Source: three-view drawing plus pictorial views. Frame: mm from the lowest corner of the part. A direction names the side the tool comes from. Coordinates: 2 decimals unless noted, no trailing zeros. Write each loop counter-clockwise with the first axis right and the second up, starting at its lowest first coordinate (ties: lowest second). Pieces come first, ordered by that corner, then holes. Notation, with made-up numbers: (10.5, -20) - (47.5, -20) arc R6 cw to (47.5, -14) - close; hole circle Ø4 at (22, 85.5). An arc over 180 degrees is marked (long way). Answer as a JSON object with one key per item and string values. Group by question number.
Item 1: Section C-C on y = 10. Return loops of the section in (x, z), and give its area (3 significant figures).
Item 2: Line query: line 1 along X through (y, z) = (13.75, 10.5); line 2 along X through (y, z) = (11.75, 22.75); line 3 along Y through (x, z) = (7.5, 10). Output: solid intervals per line, ascending. Write a range as from..to.
Item 3: Section D-D on x = 27.5. Return loops of the section in (y, z).
Item 4: Section A-A on z = 10.5. Return loops of the section in (x, y), and give its area (3 significant figures).
Item 5: Section B-B on x = 17.5. Return loops of the section in (y, z), and give its area (3 significant figures).
Item 6: First-contact query: pin 1 Ø8 at (x, y) = (7.5, 10) entering from -Z; pin 2 Ø3.5 at (x, y) = (23.5, 3) entering from +Z. Flat tips, straight axial feed; report the tip coordinate or a pass-through.
Item 7: Set-up query: the marked faces 1, 2 and 3. Return all of +Z, -Z, +X, -X, +Y, -Y with unobstructed straight access to the full face (end or side cutting, diameter ignored); none if empty.
Item 8: Mould query, pull axis X, two halves, no side actions, for the marked faces 4, 5, 6 and 7. Classes: pulls with the +X half, pulls with the -X half, needs draft (parallel to the pull), parting line crosses it, or undercut.
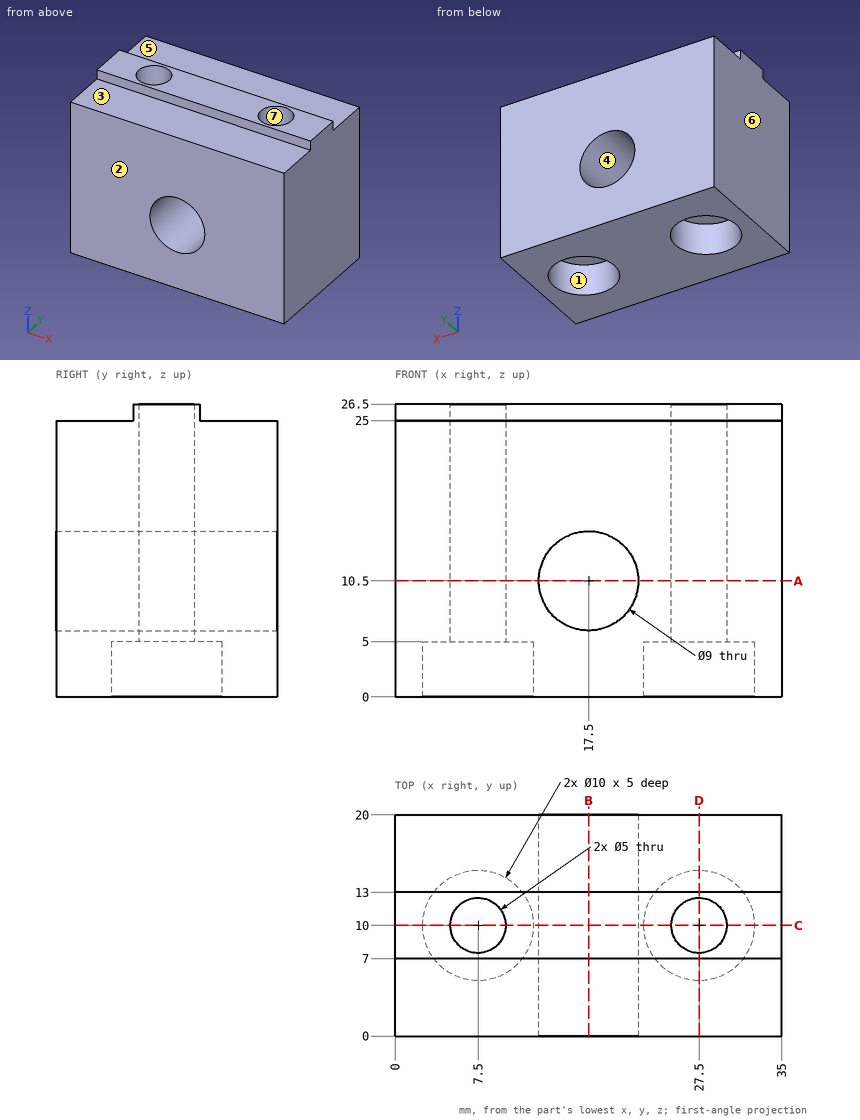
Checks:
{
 "1": {"outline": "(0, 0) - (2.5, 0) - (2.5, 5) - (5, 5) - (5, 26.5) - (0, 26.5) - close; (10, 5) - (12.5, 5) - (12.5, 0) - (22.5, 0) - (22.5, 5) - (25, 5) - (25, 26.5) - (10, 26.5) - close; (30, 5) - (32.5, 5) - (32.5, 0) - (35, 0) - (35, 26.5) - (30, 26.5) - close; hole circle Ø9 at (17.5, 10.5)", "area": "549 mm^2"},
 "2": {"line 1": "0..13, 22..35", "line 2": "0..5.71, 9.29..25.71, 29.29..35", "line 3": "0..7.5, 12.5..20"},
 "3": {"outline": "(0, 0) - (5, 0) - (5, 5) - (7.5, 5) - (7.5, 26.5) - (7, 26.5) - (7, 25) - (0, 25) - close; (12.5, 5) - (15, 5) - (15, 0) - (20, 0) - (20, 25) - (13, 25) - (13, 26.5) - (12.5, 26.5) - close"},
 "4": {"outline": "(0, 0) - (13, 0) - (13, 20) - (0, 20) - close; (22, 0) - (35, 0) - (35, 20) - (22, 20) - close; hole circle Ø5 at (7.5, 10); hole circle Ø5 at (27.5, 10)", "area": "481 mm^2"},
 "5": {"outline": "(0, 0) - (20, 0) - (20, 6) - (0, 6) - close; (0, 15) - (20, 15) - (20, 25) - (13, 25) - (13, 26.5) - (7, 26.5) - (7, 25) - (0, 25) - close", "area": "329 mm^2"},
 "6": {"pin 1": "z = 5", "pin 2": "z = 25"},
 "7": {"face 1": "-Z", "face 2": "+Z, -Z, +X, -X, -Y", "face 3": "+Z, +X, -X, -Y"},
 "8": {"face 4": "undercut", "face 5": "needs draft", "face 6": "pulls with the -X half", "face 7": "undercut"}
}
